Geometry check sheet. Reference: the model listing, model coordinates, mm. A direction names the side the tool comes from. Coordinates: 2 decimals unless noted, no trailing zeros. Loops run counter-clockwise (first coordinate to the right, second up) from the corner with the lowest first, then second, coordinate; pieces in that order, holes last. Notation, with made-up numbers: (16, 37) - (42, 37) arc R25 ccw to (42, 76) - close; hole circle Ø9 at (12.25, 87.25). An arc over 180 degrees is marked (long way). Write item = value, one per line. Start each with the question number.
from build123d import *

# Parameters (mm, degrees)
SALIENTE_EXTRUIR1_DEPTH = 18
CROQUIS2_R              = 3.4
CORTAR_EXTRUIR1_DEPTH   = 22
CROQUIS3_R              = 1.5
CORTAR_EXTRUIR2_DEPTH   = 22
CROQUIS4_W              = 1.55
CROQUIS4_H              = 2.5
CORTAR_EXTRUIR3_DEPTH   = 47.683139164
CHAFL_N1_SIZE           = 3
CROQUIS5_W              = 10
CROQUIS5_H              = 6
CORTAR_EXTRUIR4_DEPTH   = 5


with BuildPart() as part:
    # Croquis1 → Saliente-Extruir1 (new body)
    with BuildSketch(Plane.XY):
        with BuildLine():
            Line((0, -6.350148368), (0, 20.649851632))
            Line((0, 20.649851632), (-36, 20.649851632))
            Line((-36, 20.649851632), (-36, 21.649851632))
            ThreePointArc((-36, 21.649851632), (-35.414213562, 23.064065194), (-34, 23.649851632))
            Line((-34, 23.649851632), (3, 23.649851632))
            Line((3, 23.649851632), (3, -6.350148368))
            Line((3, -6.350148368), (0, -6.350148368))
        make_face()
    extrude(amount=SALIENTE_EXTRUIR1_DEPTH)

    # Croquis2 → Cortar-Extruir1 (cut)
    with BuildSketch(Plane(origin=(3, 0, 0), x_dir=(0, 0, -1), z_dir=(1, 0, 0))):
        with Locations(Location((-9, 5.649851632, 0), (0, 0, 90))):
            Circle(CROQUIS2_R)
    extrude(amount=-CORTAR_EXTRUIR1_DEPTH, mode=Mode.SUBTRACT)

    # Croquis3 → Cortar-Extruir2 (cut)
    with BuildSketch(Plane(origin=(0, 23.649851632, 0), x_dir=(1, 0, 0), z_dir=(0, 1, 0))):
        with Locations(Location((-31, -5, 0), (0, 0, 180))):
            Circle(CROQUIS3_R)
        with Locations(Location((-31, -13, 0), (0, 0, 180))):
            Circle(CROQUIS3_R)
    extrude(amount=-CORTAR_EXTRUIR2_DEPTH, mode=Mode.SUBTRACT)

    # Croquis4 → Cortar-Extruir3 (cut, through all)
    with BuildSketch(Plane.ZY):
        with BuildLine():
            Line((0, 20.999851632), (4, 16.999851632))
            Line((4, 16.999851632), (4, -1.408653875))
            ThreePointArc((4, -1.408653875), (6.37641206, -2.59267749), (9, -3.000148368))
            Line((9, -3.000148368), (18, -3.000148368))
            Line((18, -3.000148368), (18, -6.350148368))
            Line((18, -6.350148368), (0, -6.350148368))
            Line((0, -6.350148368), (0, 20.999851632))
        make_face()
        with Locations((17.225, 5.649851632)):
            Rectangle(CROQUIS4_W, CROQUIS4_H)
    extrude(amount=-CORTAR_EXTRUIR3_DEPTH, mode=Mode.SUBTRACT)

    # Chaflán1
    chafl_n1_edges = [part.edges().sort_by_distance(p)[0] for p in [
        (3, 23.649851632, 9),
        (0, 20.649851632, 9.175),
    ]]
    chamfer(chafl_n1_edges, length=CHAFL_N1_SIZE)

    # Croquis5 → Cortar-Extruir4 (cut)
    with BuildSketch(Plane(origin=(0, 23.649851632, 0), x_dir=(1, 0, 0), z_dir=(0, 1, 0))):
        with Locations((-2, -9)):
            Rectangle(CROQUIS5_W, CROQUIS5_H)
    extrude(amount=-CORTAR_EXTRUIR4_DEPTH, mode=Mode.SUBTRACT)


solid = part.part
(1) Scan lines: line 1 (Z direction, x = -31, y = 22.6); line 2 (Z direction, x = 0.5, y = -1.25); line 3 (Y direction, x = -29.5, z = 4). Record each from-to range of solid material in increasing order.
(2) Sectioned sample at B-B on x = -31. Enter the section's corners in (y, z).
(3) Draft check along X on faces 4 (the face through (-29.5, 22.17, 5.07)), 5 (the face through (-35.43, 23.05, 8.87)), 6 (the face through (1, -3, 13)). Enter one of: pulls with the +X half, pulls with the -X half, needs draft (parallel to the pull), parting line crosses it, or undercut.
(4) Tool access check on faces 1 (the face through (1, 8, 4)), 2 (the face through (-2, 22, 6)), 3 (the face through (1, 18.65, 9)). Record the directions out of +Z, -Z, +X, -X, +Y, -Y that give a thin tool (end or side, any length) a straight path to the whole face; none if there is none.
(5) Sectioned sample at D-D on y = 22.25. Enter the section's corners in (x, z), plus the area to 3 significant figures.
(6) Sectioned sample at C-C on z = 13. Enter the section's corners in (x, y), plus the area to 3 significant figures.
(7) Depth check by flat-ended pin: pin 1 (3 mm diameter, centred on x = 1, z = 8.5, fed in from +Y); pin 2 (5 mm diameter, centred on x = -20.5, z = 14, fed in from -Y); pin 3 (0.9 mm diameter, centred on y = 22, z = 8.5, fed in from +X). Enter the tip coordinate at first touch or a pass-through.
(8) Sectioned sample at A-A on x = -3.5. Enter the section's corners in (y, z), plus the area to 3 significant figures.
Working result:
q1.line_1 = 0 to 3.5, 6.5 to 11.5, 14.5 to 18
q1.line_2 = 4 to 18
q1.line_3 = 20.65 to 23.65
q2.outline = (20.65, 0) - (23.65, 0) - (23.65, 3.5) - (20.65, 3.5) - close; (20.65, 6.5) - (23.65, 6.5) - (23.65, 11.5) - (20.65, 11.5) - close; (20.65, 14.5) - (23.65, 14.5) - (23.65, 18) - (20.65, 18) - close
q3.face_4 = undercut
q3.face_5 = pulls with the -X half
q3.face_6 = needs draft
q4.face_1 = -Z, +X, -X, -Y
q4.face_2 = +X, +Y
q4.face_3 = +X, -X, +Y
q5.outline = (-35.91, 0) - (1.4, 0) - (1.4, 6) - (-7, 6) - (-7, 12) - (1.4, 12) - (1.4, 18) - (-35.91, 18) - close; hole circle Ø3 at (-31, 5); hole circle Ø3 at (-31, 13)
q5.area = 607 mm2
q6.outline = (-36, 20.65) - (-32.5, 20.65) - (-32.5, 23.65) - (-34, 23.65) arc R2 ccw to (-36, 21.65) - close; (-29.5, 20.65) - (-3, 20.65) - (0, 17.65) - (0, -3) - (3, -3) - (3, 20.65) - (0, 23.65) - (-29.5, 23.65) - close
q6.area = 178 mm2
q7.pin_1 = 18.65
q7.pin_2 = 20.65
q7.pin_3 = -7
q8.outline = (20.65, 0) - (23.65, 0) - (23.65, 6) - (20.65, 6) - close; (20.65, 12) - (23.65, 12) - (23.65, 18) - (20.65, 18) - close
q8.area = 36.0 mm2
